Here's how the part is built. I have some questions about the finished solid (model axes, mm). Face numbers are marked on the shaded views. A direction names the side the tool comes from. Round coordinates to 2 decimals unless told otherwise and drop trailing zeros. Order: outer loops, then holes, each group sorted by start corner. A loop starts at its lowest first (then second) coordinate and runs counter-clockwise, first axis right, second up. Notation, with made-up numbers: (86.25, 27) - (140.25, 27) arc R5 ccw to (140.25, 36) - close; hole circle Ø2 at (-2.75, -5). An arc over 180 degrees is marked (long way). One line per item, written item: value.
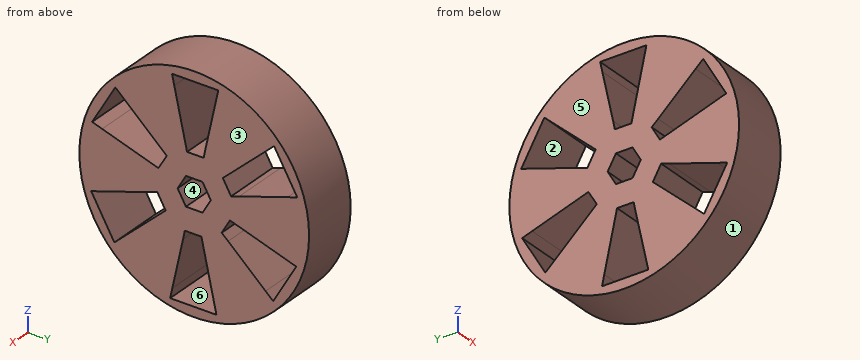
Autodesk Inventor part; units mm, degrees
ref_plane "YZ Plane" through (0, 0, 0) normal (1, 0, 0) x (0, 1, 0)
ref_plane "XZ Plane" through (0, 0, 0) normal (0, 1, 0) x (-1, 0, 0)
ref_plane "XY Plane" through (0, 0, 0) normal (0, 0, 1) x (1, 0, 0)
sketch "Sketch1" plane through (0, 0, 0) normal (1, 0, 0) x (0, 1, 0)
  circle A0 centre (0, 0) radius 50.8
  dimension "d16" = 101.6
extrude "Extrusion1" add sketch "Sketch1" along normal blind 25.4
sketch "Sketch2" plane through (25.4, 0, 0) normal (1, 0, 0) x (0, 0, -1)
  circle A0 centre (0, 0) radius 50.8
  circle A1 centre (0, 0) radius 25.4
  line L0 (6.35, 3.6662) -> (6.35, -3.6662)
  line L1 (6.35, -3.6662) -> (0, -7.3323)
  line L2 (0, -7.3323) -> (-6.35, -3.6662)
  line L3 (-6.35, -3.6662) -> (-6.35, 3.6662)
  line L4 (-6.35, 3.6662) -> (0, 7.3323)
  line L5 (0, 7.3323) -> (6.35, 3.6662)
  circle A2 centre (0, 0) radius 44.45
  line L6 (0, 0) -> (-11.3174, 49.5233)
  circle A3 centre (0, 0) radius 50.8
  line L7 (0, 0) -> (10.4532, 49.7129)
  arc A4 (9.1466, 43.4988) -> (-9.9027, 43.3329) centre (0, 0) ccw
  point P0 (5.2266, 24.8564)
  point P1 (-5.6587, 24.7616)
  dimension "d3" = 25.4
  dimension "d4" = 6.35
  dimension "d5" = 0
  dimension "d8" = 6.35
  dimension "d9" = 19.05
  dimension "d10" = 0
extrude "Extrusion4" cut sketch "Sketch2" against normal through all contours L7 L6 L4 L5 | L5 L0 L1 L2 L3 L4 L6 L7
sketch "Sketch3" plane through (25.4, 0, 0) normal (1, 0, 0) x (0, 0, -1)
  circle A0 centre (0, 0) radius 50.8
  line L0 (-46.4628, -9.6079) -> (-46.4628, 9.6097)
  line L1 (-16.4289, -3.168) -> (-41.9244, -8.8202)
  line L2 (-42.0194, 9.6834) -> (-20.1547, 4.9235)
  line L3 (-16.4289, 4.1621) -> (-16.4289, -3.168)
  line L4 (-16.4289, 4.1621) -> (-20.1547, 4.9235)
  line L5 (-42.0194, 9.6834) -> (-46.4628, 10.6507)
  line L6 (-46.4628, 10.6507) -> (-46.4628, 9.6097)
  line L7 (-41.9244, -8.8202) -> (-46.4628, -9.8264)
  line L8 (-46.4628, -9.8264) -> (-46.4628, -9.6079)
extrude "Extrusion5" cut sketch "Sketch3" against normal through all contours L0 L6 L5 L2 L4 L3 L1 L7 L8
pattern_circular "Circular Pattern2" count 6 over 360 about axis through (0, 0, 0) along (1, 0, 0) of "Extrusion5"
properties part number "part_4 in. Compliance Wheel" material "ABS Plastic"
Q1. If I drill on line 1 along Y through (x, z) = (6.25, -20); line 2 along Z through (x, y) = (23, 33.5); line 3 along Z through (x, y) = (10, -33), over which ranges is the centre line in solid material (lowest first)?
Results list:
line 1: -46.7 to -42.1, -22.51 to -4.89, 3.96 to 21.22, 42.1 to 46.7
line 2: -38.19 to -31.17, -11.05 to 10.15, 30.07 to 38.19
line 3: -38.62 to -29.61, -9.99 to 10.89, 30.72 to 38.62
Q2. If we section it at C-C, the plane x = 5: Give the number of separate pieces and of enclosed holes in the cut face, then the cut area to 3 significant figures.
Results list:
separate pieces: 1
enclosed holes: 7
area: 5,470 mm²
Q3. We'd pull the mould along Y, two halves only. Please class the marked faces 1, 2, 3 and 4: released by +Y, released by -Y, zero draft, split by the parting line, or undercut.
Results list:
face 1: split by the parting line
face 2: undercut
face 3: zero draft
face 4: undercut
Q4. If we section it at A-A, the plane y = 0: Please give me the cut outline in (x, z).
Results list:
outline: (0, -50.8) - (25.4, -50.8) - (25.4, -46.46) - (0, -46.46) - close; (0, -16.43) - (25.4, -16.43) - (25.4, -6.35) - (0, -6.35) - close; (0, 6.35) - (25.4, 6.35) - (25.4, 16.43) - (0, 16.43) - close; (0, 46.46) - (25.4, 46.46) - (25.4, 50.8) - (0, 50.8) - close
Q5. Will these pins go through, and if not, where does the flat tip stop? pin 1 (10 mm diameter, centred on x = 3.5, y = 9.5, fed in from -Z); pin 2 (5 mm diameter, centred on x = 17.5, z = -22, fed in from -Y); pin 3 (6 mm diameter, centred on x = 13.5, z = -22.5, fed in from +Y).
Results list:
pin 1: z = -50.6
pin 2: y = -46.91
pin 3: y = 46.91
Q6. Which directions (+Z, -Z, +X, -X, +Y, -Y) give clear straight access to the entire face, cutting with the end or side of a thin tool? Please do the marked faces 5 and 6.
Results list:
face 5: +Z, -Z, -X, +Y, -Y
face 6: +X, -X
Q7. If we section it at B-B, the plane z = -37.5: Please give me the cut outline in (x, y), then the cut area to 3 significant figures.
Results list:
outline: (0, -34.27) - (25.4, -34.27) - (25.4, -8.7) - (0, -8.7) - close; (0, 7.84) - (25.4, 7.84) - (25.4, 34.27) - (0, 34.27) - close
area: 1,320 mm²
